Check sheet for the modelled part. Datum: model origin and axes. Units: mm. A direction names the side the tool comes from. Give positions to 0.01 mm unless a question says otherwise; leave off trailing zeros. Order: outer loops, then holes, each group sorted by start corner. A loop starts at its lowest first (then second) coordinate and runs counter-clockwise, first axis right, second up. Notation, with made-up numbers: (68, 5) -> (81, 5) arc R20 ccw to (81, 9) -> close; hole circle Ø1 at (74, 10). An arc over 180 degrees is marked (long way). Write each question's results on one line, items separated by ' | '.
from build123d import *

# Parameters (mm, degrees)
SKETCH_1_R               = 21
EXTRUDE_1_DEPTH          = 26
SKETCH_2_R               = 14
EXTRUDE_2_DEPTH          = 15
EXTRUDE_3_DEPTH          = 16
SKETCH_5_R               = 3.1
EXTRUDE_4_DEPTH          = 14.5
SKETCH_6_R               = 17
CUT_EXTRUDE_2_DEPTH      = 16
SKETCH_7_R               = 9
CUT_EXTRUDE_3_DEPTH      = 4
SKETCH_8_R               = 6.25
CUT_EXTRUDE_4_DEPTH      = 50.658836072
CUT_EXTRUDE_START        = -4
SKETCH_9_R               = 9
CUT_EXTRUDE_5_DEPTH      = 4
CUT_EXTRUDE_6_REACH      = 80.045
CUT_EXTRUDE_6_END_RADIUS = 17
SKETCH_10_R              = 1.75
HOLE_WIZARD_M5_1_REACH   = 76.155
HOLE_WIZARD_M5_1_BORE_R  = 2.1


with BuildPart() as part:
    # 草图1 → 凸台-拉伸1 (new body)
    with BuildSketch(Plane(origin=(0, 0, 0), x_dir=(0, 0, -1), z_dir=(1, 0, 0))):
        with Locations(Location((0, 0, 0), (0, 0, 180))):
            Circle(SKETCH_1_R)
    extrude(amount=EXTRUDE_1_DEPTH)

    # 草图2 → 凸台-拉伸2 (add)
    with BuildSketch(Plane(origin=(26, 0, 0), x_dir=(0, 0, -1), z_dir=(1, 0, 0))):
        Circle(SKETCH_2_R)
    extrude(amount=EXTRUDE_2_DEPTH)

    # 草图4 → 凸台-拉伸3 (add)
    with BuildSketch(Plane.ZY):
        with BuildLine():
            Line((0, 27), (-8.5, 27))
            Line((-8.5, 27), (-18.109583017, 10.63216831))
            ThreePointArc((-18.109583017, 10.63216831), (-10.433706568, 18.224647246), (0, 21))
            Line((0, 21), (0, 27))
        make_face()
        with BuildLine():
            Line((8.5, 27), (0, 27))
            Line((0, 27), (0, 21))
            ThreePointArc((0, 21), (10.433706568, 18.224647246), (18.109583017, 10.63216831))
            Line((18.109583017, 10.63216831), (8.5, 27))
        make_face()
    extrude(amount=-EXTRUDE_3_DEPTH)

    # 草图5 → 凸台-拉伸4 (add, symmetric)
    with BuildSketch(Plane.XY):
        with BuildLine():
            Line((16, -14), (0, -14))
            Line((0, -14), (0, -21.041445119))
            Line((0, -21.041445119), (-5.007077172, -25.534204154))
            ThreePointArc((-5.007077172, -25.534204154), (-6.479163396, -27.554847963), (-7, -30))
            ThreePointArc((-7, -30), (-3.575969226, -35.418891265), (2.788127515, -34.652965713))
            Line((2.788127515, -34.652965713), (16, -23.896759721))
            Line((16, -23.896759721), (16, -14))
        make_face()
        with Locations(Location((-1, -30, 0), (0, 0, 180))):
            Circle(SKETCH_5_R, mode=Mode.SUBTRACT)
    extrude(amount=EXTRUDE_4_DEPTH, both=True)

    # 草图6 → 切除-拉伸2 (cut)
    with BuildSketch(Plane.ZY):
        Circle(SKETCH_6_R)
    extrude(amount=-CUT_EXTRUDE_2_DEPTH, mode=Mode.SUBTRACT)

    # 草图7 → 切除-拉伸3 (cut)
    with BuildSketch(Plane.ZY.offset(-16)):
        Circle(SKETCH_7_R)
    extrude(amount=-CUT_EXTRUDE_3_DEPTH, mode=Mode.SUBTRACT)

    # 草图8 → 切除-拉伸4 (cut, through all)
    with BuildSketch(Plane.ZY.offset(-20)):
        Circle(SKETCH_8_R)
    extrude(amount=-CUT_EXTRUDE_4_DEPTH, mode=Mode.SUBTRACT)

    # 草图9 → 切除-拉伸5 (cut)
    with BuildSketch(Plane(origin=(41, 0, 0), x_dir=(0, 0, -1), z_dir=(1, 0, 0)).offset(CUT_EXTRUDE_START)):
        with Locations(Location((0, 0, 0), (0, 0, 180))):
            Circle(SKETCH_9_R)
    extrude(amount=CUT_EXTRUDE_5_DEPTH, mode=Mode.SUBTRACT)

    # 切除-拉伸6: up to this cylinder (the profile starts outside it)
    cut_extrude_6_end = Plane(origin=(8, 0, 0), z_dir=(-1, 0, 0)) * Cylinder(CUT_EXTRUDE_6_END_RADIUS, 195.09, mode=Mode.PRIVATE)
    # 草图10 → 切除-拉伸6 (cut, up to the surface)
    with BuildSketch(Plane(origin=(0, 27, 0), x_dir=(1, 0, 0), z_dir=(0, 1, 0)), mode=Mode.PRIVATE) as cut_extrude_6_sk1:
        with Locations(Location((8, 0, 0), (0, 0, 270))):
            Circle(SKETCH_10_R)
    cut_extrude_6_tool1 = extrude(cut_extrude_6_sk1.sketch, amount=-CUT_EXTRUDE_6_REACH, mode=Mode.PRIVATE) - cut_extrude_6_end
    add(cut_extrude_6_tool1.solids().sort_by_distance((8, 27, 0))[0], mode=Mode.SUBTRACT)

    # M5 螺纹孔1 bore (on position points) → M5 螺纹孔1 (cut, up to next)
    with BuildSketch(Plane(origin=(8, 27, 0), x_dir=(0, 0, 1), z_dir=(0, 1, 0)), mode=Mode.PRIVATE) as hole_wizard_m5_1_sk1:
        Circle(HOLE_WIZARD_M5_1_BORE_R)
    hole_wizard_m5_1_tool1 = extrude(hole_wizard_m5_1_sk1.sketch, amount=-HOLE_WIZARD_M5_1_REACH, mode=Mode.PRIVATE) & part.part
    add(hole_wizard_m5_1_tool1.solids().sort_by_distance((8, 27, 0))[0], mode=Mode.SUBTRACT)


solid = part.part
1. Mould release check, pull along Y, two halves, no side actions. Record for faces 1 (the flat face through (37, 1.87, -6.13)), 2 (the flat face through (26, 14, 4)), 3 (the flat face through (10, 27, 2)): +Y half, -Y half, draft (parallel to the pull), parting line (faces both ways), or undercut.
Verdict:
face 1: undercut | face 2: draft | face 3: +Y half
2. Section check D-D on y = 19.5. Record the cut outline in (x, z), then the cut area to 3 significant figures.
Verdict:
outline: (0, -12.9) -> (16, -12.9) -> (16, -7.79) -> (26, -7.79) -> (26, 7.79) -> (16, 7.79) -> (16, 12.9) -> (0, 12.9) -> close; hole circle Ø4.2 at (8, 0) | area: 555 mm^2
3. Section check C-C on x = -1. Record the cut outline in (y, z), then the cut area to 3 significant figures.
Verdict:
outline: (-36, -14.5) -> (-33.1, -14.5) -> (-33.1, 14.5) -> (-36, 14.5) -> close; (-26.9, -14.5) -> (-21.94, -14.5) -> (-21.94, 14.5) -> (-26.9, 14.5) -> close | area: 228 mm^2
4. Section check A-A on y = 0. Record the cut outline in (x, z).
Verdict:
outline: (0, -21) -> (26, -21) -> (26, -14) -> (41, -14) -> (41, -9) -> (37, -9) -> (37, -6.25) -> (20, -6.25) -> (20, -9) -> (16, -9) -> (16, -17) -> (0, -17) -> close; (0, 17) -> (16, 17) -> (16, 9) -> (20, 9) -> (20, 6.25) -> (37, 6.25) -> (37, 9) -> (41, 9) -> (41, 14) -> (26, 14) -> (26, 21) -> (0, 21) -> close
5. Access from +Z, -Z, +X, -X, +Y, -Y to the whole of each face (thin tool, end or side, straight path). Record for faces 4 (the flat face through (0, 17.1, 1.5)), 5 (the flat face through (4, -23, -14.5)), 6 (the cylindrical face through (17.972, 8.923, -1.172)), 7 (the cylindrical face through (10.082, 22.004, -0.273)).
Verdict:
face 4: +Z, -Z, -X, +Y | face 5: -Z, +X, -X, -Y | face 6: -X | face 7: +Y
6. Material ranges on probe 1 along X at (y, z) = (24, 0); probe 2 along Y at (x, z) = (38.5, 0); probe 3 along X at (y, z) = (10, -15), recorded low to high. Write a range as from..to.
Verdict:
probe 1: x = 0..5.9, 10.1..16 | probe 2: y = -14..-9, 9..14 | probe 3: x = 0..26
7. Gauge pin test, flat ends, axial feed: pin 1 Ø1 at (x, z) = (15, -7) entering from -Y; pin 2 Ø10 at (x, y) = (1, 10.5) entering from -Z; pin 3 Ø5.5 at (y, z) = (2, -4) entering from -X; pin 4 Ø23.5 at (y, z) = (0, 0) entering from +X. Record the tip position at first contact, or that the pin passes through.
Verdict:
pin 1: stops at y = -25.12 | pin 2: stops at z = -20.27 | pin 3: stops at x = 20 | pin 4: stops at x = 41
8. Section check B-B on z = 0. Give the number of separate pieces and of enclosed holes in the cut face, then the cut area to 3 significant figures.
Verdict:
separate pieces: 3 | enclosed holes: 1 | area: 859 mm^2
